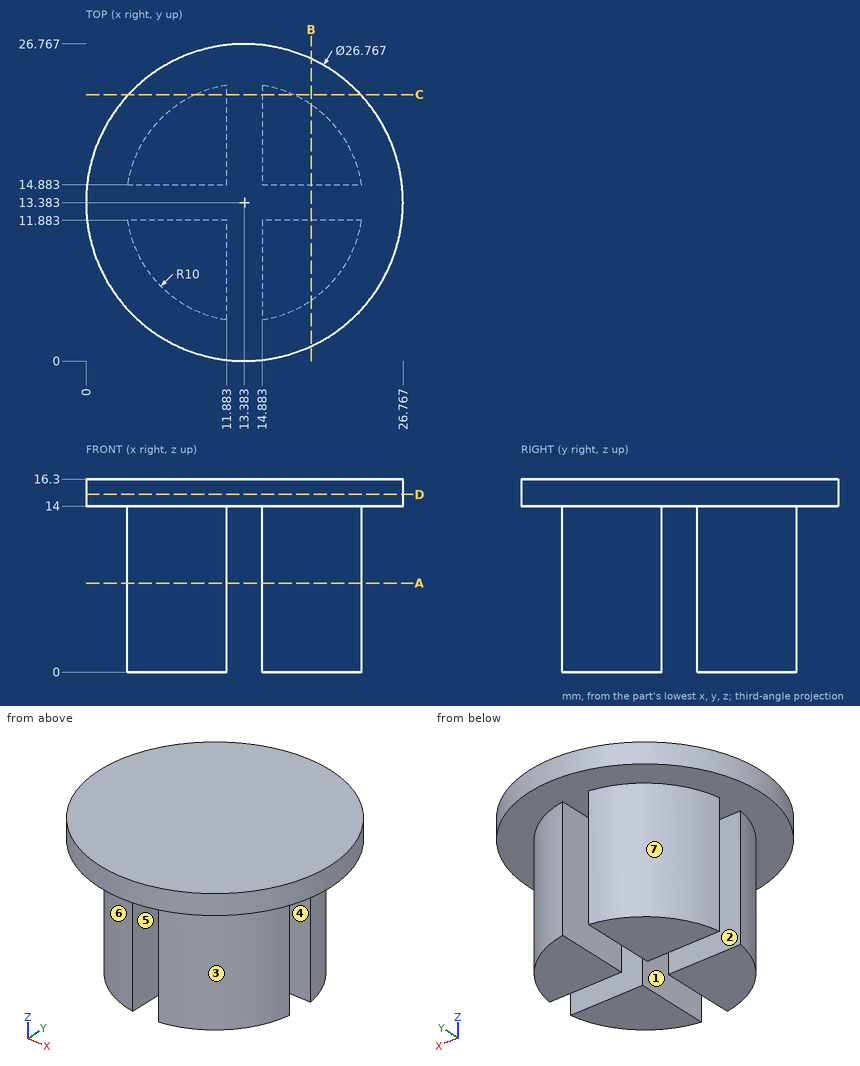
Can you work these out from the drawing? Everything is in mm from the part's minimum corner. A direction names the side the tool comes from. Round coordinates to 2 decimals unless told otherwise and drop trailing zeros. Loops run counter-clockwise (first coordinate to the right, second up) from the corner with the lowest first, then second, coordinate; pieces in that order, holes last. Notation, with made-up numbers: (-12, 3) -> (34, 3) arc R37 cw to (34, 41) -> close; hole circle Ø5 at (31, -2). An arc over 180 degrees is marked (long way). Answer in a Markdown table with one row per item.
Item 1: Suppose I cut it at C-C, the plane y = 22.5. List the corners of the cut face in (x, z) for me (1 decimal).
Answer block:
| item | result |
|---|---|
| outline | (3.6, 14) -> (9.3, 14) -> (9.3, 0) -> (11.9, 0) -> (11.9, 14) -> (14.9, 14) -> (14.9, 0) -> (17.5, 0) -> (17.5, 14) -> (23.2, 14) -> (23.2, 16.3) -> (3.6, 16.3) -> close |
Item 2: We'd pull the mould along Y, two halves only. Please class the marked faces 1, 2 and 3: released by +Y, released by -Y, zero draft, split by the parting line, or undercut.
Answer block:
| item | result |
|---|---|
| face 1 | zero draft |
| face 2 | undercut |
| face 3 | released by -Y |
Item 3: On a 3-axis mill with a long thin cutter (end or side, diameter ignored), from which of +Z, -Z, +X, -X, +Y, -Y can I reach the whole of each face in a straight line? I mean the marked faces 4, 5, 6 and 7. Say none if no direction works.
Answer block:
| item | result |
|---|---|
| face 4 | -Z, +X, -X |
| face 5 | -Z, +Y, -Y |
| face 6 | -Z, -X, -Y |
| face 7 | -Z, -X, +Y |
Item 4: Suppose I cut it at A-A, the plane z = 7.5. List the corners of the cut face in (x, y) for me.
Answer block:
| item | result |
|---|---|
| outline | (3.5, 11.88) arc R10 ccw to (11.88, 3.5) -> (11.88, 11.88) -> close; (3.5, 14.88) -> (11.88, 14.88) -> (11.88, 23.27) arc R10 ccw to start; (14.88, 3.5) arc R10 ccw to (23.27, 11.88) -> (14.88, 11.88) -> close; (14.88, 14.88) -> (23.27, 14.88) arc R10 ccw to (14.88, 23.27) -> close |
Item 5: Suppose I cut it at D-D, the plane z = 15. List the corners of the cut face in (x, y) for me.
Answer block:
| item | result |
|---|---|
| outline | circle Ø26.77 at (13.38, 13.38) |
Item 6: Suppose I cut it at B-B, the plane x = 19. List the corners of the cut face in (y, z) for me (1 decimal).
Answer block:
| item | result |
|---|---|
| outline | (1.2, 14) -> (5.1, 14) -> (5.1, 0) -> (11.9, 0) -> (11.9, 14) -> (14.9, 14) -> (14.9, 0) -> (21.7, 0) -> (21.7, 14) -> (25.5, 14) -> (25.5, 16.3) -> (1.2, 16.3) -> close |
Item 7: If I drill on probe 1 along Z at (x, y) = (12, 12); probe 2 along X at (y, z) = (13, 15.25) (1 decimal); probe 3 along Y at (x, z) = (21, 9.25) (1 decimal), over which ranges is the centre line in solid material (lowest first)?
Answer block:
| item | result |
|---|---|
| probe 1 | 14 to 16.3 |
| probe 2 | 0 to 26.8 |
| probe 3 | 6.9 to 11.9, 14.9 to 19.9 |
Item 8: Will these pins go through, and if not, where does the flat tip stop? P1, Ø6.5, axis at x = 6.5, z = 9, coming from the +Y side; P2, Ø8, axis at x = 17, y = 11, coming from the -Z side; P3, Ø6.5, axis at y = 7.5, z = 4, coming from the -X side; P4, Ø5, axis at x = 22, z = 5.5, coming from the -Y side.
Answer block:
| item | result |
|---|---|
| P1 | y = 22.7 |
| P2 | z = 0 |
| P3 | x = 3.74 |
| P4 | y = 5.47 |
